Could you check a few things on this model? Use its own coordinates, in mm. A direction names the side the tool comes from. Coordinates: 2 decimals unless noted, no trailing zeros. Order: outer loops, then holes, each group sorted by start corner. A loop starts at its lowest first (then second) coordinate and runs counter-clockwise, first axis right, second up. Notation, with made-up numbers: M -2,45 L 48,45 A23 ccw 48,81 Z; hole C 26,87.5 d10. An arc over 180 degrees is marked long. One line per question, with ' | ' between items. Start each with the question number.
from build123d import *

# Parameters (mm, degrees)
EXTRUDE_1_DEPTH     = 34.5
SKETCH_4_W          = 41.6
SKETCH_4_H          = 29.6
CUT_EXTRUDE_1_DEPTH = 5
EXTRUDE_2_DEPTH     = 3
SKETCH_6_W          = 5.4
SKETCH_6_H          = 1.5
CUT_EXTRUDE_2_DEPTH = 57.250955547
SKETCH_7_R          = 1.22
SKETCH_7_R_2        = 0.91
SKETCH_7_R_3        = 1.3
SKETCH_7_R_4        = 1.68
SKETCH_7_R_5        = 0.95
SKETCH_7_R_6        = 0.85
CUT_EXTRUDE_3_DEPTH = 44.200115741


with BuildPart() as part:
    # 草圖1 → 填料-伸長1 (new body)
    with BuildSketch(Plane(origin=(0, 0, 0), x_dir=(1, 0, 0), z_dir=(0, 1, 0))):
        with BuildLine():
            Line((-10, -15.6), (10, -15.6))
            ThreePointArc((10, -15.6), (17.636753237, -12.436753237), (20.8, -4.8))
            Line((20.8, -4.8), (20.8, 4.8))
            ThreePointArc((20.8, 4.8), (17.636753237, 12.436753237), (10, 15.6))
            Line((10, 15.6), (-10, 15.6))
            ThreePointArc((-10, 15.6), (-17.636753237, 12.436753237), (-20.8, 4.8))
            Line((-20.8, 4.8), (-20.8, -4.8))
            ThreePointArc((-20.8, -4.8), (-17.636753237, -12.436753237), (-10, -15.6))
        make_face()
        with BuildLine():
            Line((-10, -14.8), (10, -14.8))
            ThreePointArc((10, -14.8), (17.071067812, -11.871067812), (20, -4.8))
            Line((20, -4.8), (20, 4.8))
            ThreePointArc((20, 4.8), (17.071067812, 11.871067812), (10, 14.8))
            Line((10, 14.8), (-10, 14.8))
            ThreePointArc((-10, 14.8), (-17.071067812, 11.871067812), (-20, 4.8))
            Line((-20, 4.8), (-20, -4.8))
            ThreePointArc((-20, -4.8), (-17.071067812, -11.871067812), (-10, -14.8))
        make_face(mode=Mode.SUBTRACT)
    extrude(amount=EXTRUDE_1_DEPTH)

    # 草圖4 → 除料-伸長1 (cut)
    with BuildSketch(Plane(origin=(0, 34.5, 0), x_dir=(1, 0, 0), z_dir=(0, 1, 0))):
        Rectangle(SKETCH_4_W, SKETCH_4_H)
    extrude(amount=-CUT_EXTRUDE_1_DEPTH, mode=Mode.SUBTRACT)

    # 草圖5 → 填料-伸長2 (add)
    with BuildSketch(Plane.XZ):
        with BuildLine():
            Line((20, 4.8), (20, -4.8))
            ThreePointArc((20, -4.8), (17.071067812, -11.871067812), (10, -14.8))
            Line((10, -14.8), (-10, -14.8))
            ThreePointArc((-10, -14.8), (-17.071067812, -11.871067812), (-20, -4.8))
            Line((-20, -4.8), (-20, 4.8))
            ThreePointArc((-20, 4.8), (-17.071067812, 11.871067812), (-10, 14.8))
            Line((-10, 14.8), (10, 14.8))
            ThreePointArc((10, 14.8), (17.071067812, 11.871067812), (20, 4.8))
        make_face()
    extrude(amount=-EXTRUDE_2_DEPTH)

    # 草圖6 → 除料-伸長2 (cut, through all)
    with BuildSketch(Plane(origin=(20.8, 0, 0), x_dir=(0, 0, -1), z_dir=(1, 0, 0))):
        with Locations((0.2, 3.75)):
            Rectangle(SKETCH_6_W, SKETCH_6_H)
    extrude(amount=-CUT_EXTRUDE_2_DEPTH, mode=Mode.SUBTRACT)

    # 草圖7 → 除料-伸長3 (cut, through all)
    with BuildSketch(Plane.XZ):
        with Locations(Location((0, 0, 0), (0, 0, 270))):
            Circle(SKETCH_7_R)
        with Locations(Location((4, 0, 0), (0, 0, 270))):
            Circle(SKETCH_7_R_2)
        with Locations(Location((8, 0, 0), (0, 0, 270))):
            Circle(SKETCH_7_R_3)
        with Locations(Location((-4, 0, 0), (0, 0, 270))):
            Circle(SKETCH_7_R_2)
        with Locations(Location((-8, 0, 0), (0, 0, 270))):
            Circle(SKETCH_7_R_4)
        with Locations(Location((-12, 0, 0), (0, 0, 270))):
            Circle(SKETCH_7_R_5)
        with Locations(Location((12, 0, 0), (0, 0, 270))):
            Circle(SKETCH_7_R_6)
    extrude(amount=-CUT_EXTRUDE_3_DEPTH, mode=Mode.SUBTRACT)


solid = part.part
(1) Imagine slicing it at C-C, the plane y = 3.5. Write out the boundary of the cut face in (x, z).
(2) Imagine slicing it at A-A, the plane x = 8. Write out the boundary of the cut face in (y, z), plus the area to 3 significant figures.
(3) Imagine slicing it at B-B, the plane y = 21. Write out the boundary of the cut face in (x, z), plus the area to 3 significant figures.
(4) Imagine slicing it at D-D, the plane x = 0. Write out the boundary of the cut face in (y, z), plus the area to 3 significant figures.
(5) On a 3-axis mill with a long thin cutter (end or side, diameter ignored), from which of +Z, -Z, +X, -X, +Y, -Y can I reach the whole of each face in a straight line? I mean faces 1 (the flat face through (20, 16, 0)), 2 (the cylindrical face through (4.767, 1.479, -0.489)). Say none if no direction works.
(6) We'd pull the mould along X, two halves only. Please class faces 3 (the cylindrical face through (6.847, 1.479, -0.6)), 4 (the flat face through (20.2, 29.5, -0.1)), 5 (the flat face through (20.8, 15, 0)): +X half, -X half, draft (parallel to the pull), parting line (faces both ways), or undercut.
(7) If I drill on line 1 along Z through (x, y) = (10, 30); line 2 along X through (y, z) = (10.5, 1.5); line 3 along Y through (x, z) = (-9.5, -2), over which ranges is the centre line in solid material (lowest first)? Write a range as from..to.
(8) For P1, Ø12, axis at x = -13.5, z = -4, coming from the +Y side; P2, Ø4, axis at x = 0, z = 0, coming from the -Y side; P3, Ø12, axis at y = 15, z = 12, coming from the -X side; P4, Ø12, axis at x = 16, z = -0.5, coming from the +Y side, each with a flat end and sliding along its axis, tell me the tip position at first contact or that it passes through.
Answers:
1) outline: M -20.8,-4.8 A10.8 ccw -10,-15.6 L 10,-15.6 A10.8 ccw 20.8,-4.8 L 20.8,-2.9 L 20,-2.9 L 20,-4.8 A10 cw 10,-14.8 L -10,-14.8 A10 cw -20,-4.8 L -20,-2.9 L -20.8,-2.9 Z; M -20.8,2.5 L -20,2.5 L -20,4.8 A10 cw -10,14.8 L 10,14.8 A10 cw 20,4.8 L 20,2.5 L 20.8,2.5 L 20.8,4.8 A10.8 ccw 10,15.6 L -10,15.6 A10.8 ccw -20.8,4.8 Z
2) outline: M 0,-15.6 L 34.5,-15.6 L 34.5,-14.8 L 3,-14.8 L 3,-1.3 L 0,-1.3 Z; M 0,1.3 L 3,1.3 L 3,14.8 L 34.5,14.8 L 34.5,15.6 L 0,15.6 Z | area: 136 mm²
3) outline: M -20.8,-4.8 A10.8 ccw -10,-15.6 L 10,-15.6 A10.8 ccw 20.8,-4.8 L 20.8,4.8 A10.8 ccw 10,15.6 L -10,15.6 A10.8 ccw -20.8,4.8 Z; hole M -20,-4.8 A10 ccw -10,-14.8 L 10,-14.8 A10 ccw 20,-4.8 L 20,4.8 A10 ccw 10,14.8 L -10,14.8 A10 ccw -20,4.8 Z | area: 99.6 mm²
4) outline: M 0,-15.6 L 34.5,-15.6 L 34.5,-14.8 L 3,-14.8 L 3,-1.22 L 0,-1.22 Z; M 0,1.22 L 3,1.22 L 3,14.8 L 34.5,14.8 L 34.5,15.6 L 0,15.6 Z | area: 137 mm²
5) face 1: +Y | face 2: +Y, -Y
6) face 3: undercut | face 4: draft | face 5: +X half
7) line 1: -15.6..-14.8, 14.8..15.6 | line 2: -20.8..-20, 20..20.8 | line 3: 0..3
8) P1: y = 3 | P2: y = 0 | P3: x = -20.73 | P4: y = 29.5
